Can you work these out from the model? Positions are in its coordinate system, mm. A direction names the side the tool comes from. Round coordinates to 2 decimals unless told otherwise and drop trailing zeros. Loops run counter-clockwise (first coordinate to the right, second up) from the corner with the lowest first, then second, coordinate; pieces in that order, holes last. Notation, with made-up numbers: (15.5, -5) -> (66.5, -5) arc R21 ccw to (66.5, 4) -> close; hole circle Ø11 at (-29.5, 15). An arc over 180 degrees is marked (long way). Write each question's results on one line, items separated by ' | '.
from build123d import *

# Parameters (mm, degrees)
F1_DEPTH = 12.7
F2_W     = 6.35
F2_H     = 25.4
F3_DEPTH = 12.7
F5_DEPTH = 12.7
F6_R     = 6.35
F7_DEPTH = 12.7


with BuildPart() as f1:
    # F0 (on Right) → F1 (new body)
    with BuildSketch(Plane.YZ):
        Polygon((-25.4, 0), (0, 0), (0, 25.4), (-25.4, 25.4), (-25.4, 19.05), (-19.05, 19.05), (-19.05, 6.35), (-25.4, 6.35), align=None)
    extrude(amount=F1_DEPTH)

    # F2 (on face) → F3 (join)
    with BuildSketch(Plane(origin=(0, 0, 0), x_dir=(-1, 0, 0), z_dir=(0, 1, 0))):
        with Locations((-15.875, 12.7)):
            Rectangle(F2_W, F2_H)
    extrude(amount=-F3_DEPTH)

    # F4 (on face) → F5 (join)
    with BuildSketch(Plane(origin=(0, 0, 0), x_dir=(-1, 0, 0), z_dir=(0, 1, 0))):
        with BuildLine():
            Line((-19.05, 0), (-19.05, 25.4))
            ThreePointArc((-19.05, 25.4), (-31.75, 12.7), (-19.05, 0))
        make_face()
    extrude(amount=-F5_DEPTH)

    # F6 (on face) → F7 (cut)
    with BuildSketch(Plane(origin=(0, 0, 0), x_dir=(-1, 0, 0), z_dir=(0, 1, 0))):
        with Locations((-19.05, 12.7)):
            Circle(F6_R)
    extrude(amount=-F7_DEPTH, mode=Mode.SUBTRACT)


solid = f1.part
1. Please list where these lines run through material, in increasing order: line 1 (Z direction, x = 19.05, y = -3); line 2 (Z direction, x = 17, y = -5.75); line 3 (X direction, y = -4, z = 7.75). Write a range as from..to.
Final values:
line 1: 0..6.35, 19.05..25.4 | line 2: 0..6.69, 18.71..25.4 | line 3: 0..15.07, 23.03..30.75
2. On a 3-axis mill with a long thin cutter (end or side, diameter ignored), from which of +Z, -Z, +X, -X, +Y, -Y can I reach the whole of each face in a straight line? I mean faces 1 (the face through (6, -22, 6.35)), 2 (the face through (6, -25.4, 22)), 3 (the face through (12.7, -18, 13)). Say none if no direction works.
Final values:
face 1: +X, -X, -Y | face 2: +Z, -Z, +X, -X, -Y | face 3: +Z, -Z, +X, -Y
3. If we section it at B-B (y = -3): List the corners of the cut face in (x, z) for me.
Final values:
outline: (0, 0) -> (19.05, 0) arc R12.7 ccw to (19.05, 25.4) -> (0, 25.4) -> close; hole circle Ø12.7 at (19.05, 12.7)
4. If we section it at C-C (x = 7): List the corners of the cut face in (y, z) for me, then the cut area to 3 significant figures.
Final values:
outline: (-25.4, 0) -> (0, 0) -> (0, 25.4) -> (-25.4, 25.4) -> (-25.4, 19.05) -> (-19.05, 19.05) -> (-19.05, 6.35) -> (-25.4, 6.35) -> close | area: 565 mm2
5. If we section it at D-D (x = 24): List the corners of the cut face in (y, z) for me.
Final values:
outline: (-12.7, 1) -> (0, 1) -> (0, 8.72) -> (-12.7, 8.72) -> close; (-12.7, 16.68) -> (0, 16.68) -> (0, 24.4) -> (-12.7, 24.4) -> close
6. Will these pins go through, and if not, where does the flat tip stop? pin 1 (4 mm diameter, centred on y = -13.5, z = 5, fed in from +X); pin 2 (4 mm diameter, centred on x = 7, z = 13.5, fed in from -Y).
Final values:
pin 1: x = 30.31 | pin 2: y = -19.05
7. We'd pull the mould along Z, two halves only. Please class faces 4 (the face through (8, -13, 25.4)), 5 (the face through (6, -22, 19.05)), 6 (the face through (27, -12.7, 13)): pulls with the +Z half, pulls with the -Z half, needs draft (parallel to the pull), parting line crosses it, or undercut.
Final values:
face 4: pulls with the +Z half | face 5: undercut | face 6: needs draft
8. If we section it at A-A (z = 14.75): List the corners of the cut face in (x, y) for me, then the cut area to 3 significant figures.
Final values:
outline: (0, -19.05) -> (12.7, -19.05) -> (12.7, -12.7) -> (13.04, -12.7) -> (13.04, 0) -> (0, 0) -> close; (25.06, -12.7) -> (31.58, -12.7) -> (31.58, 0) -> (25.06, 0) -> close | area: 329 mm2
